```python
from build123d import *

# Parameters (mm, degrees)
SKETCH1_R             = 1.60655
BOSS_EXTRUDE1_DEPTH   = 0.83
BOSS_EXTRUDE4_START   = 13.5
SKETCH3_R             = 1.5
BOSS_EXTRUDE4_DEPTH   = 0.83
BOSS_EXTRUDE5_START   = -12.67
SKETCH3_5_R           = 1.5
BOSS_EXTRUDE5_DEPTH   = 0.83
BODY_MOVE_COPY1_ANGLE = 180


with BuildPart() as part:
    # Sketch1 → Boss-Extrude1 (new body)
    with BuildSketch(Plane(origin=(0, 0, 0), x_dir=(1, 0, 0), z_dir=(0, 1, 0))):
        with BuildLine():
            Line((13.5, -4.5), (13.5, 10))
            Line((13.5, 10), (8.75, 10))
            ThreePointArc((8.75, 10), (0, 7.25), (-8.75, 10))
            Line((-8.75, 10), (-13.5, 10))
            Line((-13.5, 10), (-13.5, -4.5))
            ThreePointArc((-13.5, -4.5), (-7.288689869, -8.572238768), (0, -10))
            ThreePointArc((0, -10), (7.288689869, -8.572238768), (13.5, -4.5))
        make_face()
        with Locations(Location((-7.25, 0, 0), (0, 0, 90))):
            Circle(SKETCH1_R, mode=Mode.SUBTRACT)
        with Locations(Location((7.25, 0, 0), (0, 0, 90))):
            Circle(SKETCH1_R, mode=Mode.SUBTRACT)
    extrude(amount=BOSS_EXTRUDE1_DEPTH)

    # Sketch3 → Boss-Extrude4 (add)
    with BuildSketch(Plane(origin=(0, 0, 0), x_dir=(0, 0, -1), z_dir=(1, 0, 0)).offset(BOSS_EXTRUDE4_START)):
        with BuildLine():
            Line((-4.5, 0.83), (10, 0.83))
            Line((10, 0.83), (11.5, 0.83))
            Line((11.5, 0.83), (11.5, 2.455))
            ThreePointArc((11.5, 2.455), (16.261860542, 10.323052182), (7.082672814, 10.892326816))
            ThreePointArc((7.082672814, 10.892326816), (2.026582548, 6.580128686), (-4.5, 5.33))
            Line((-4.5, 5.33), (-4.5, 0.83))
        make_face()
        with Locations((11.5, 7.83)):
            Circle(SKETCH3_R, mode=Mode.SUBTRACT)
    extrude(amount=-BOSS_EXTRUDE4_DEPTH)

    # Sketch3<5> → Boss-Extrude5 (add)
    with BuildSketch(Plane(origin=(0, 0, 0), x_dir=(0, 0, -1), z_dir=(1, 0, 0)).offset(BOSS_EXTRUDE5_START)):
        with BuildLine():
            Line((-4.5, 0.83), (10, 0.83))
            Line((10, 0.83), (11.5, 0.83))
            Line((11.5, 0.83), (11.5, 2.455))
            ThreePointArc((11.5, 2.455), (16.261860542, 10.323052182), (7.082672814, 10.892326816))
            ThreePointArc((7.082672814, 10.892326816), (2.026582548, 6.580128686), (-4.5, 5.33))
            Line((-4.5, 5.33), (-4.5, 0.83))
        make_face()
        with Locations((11.5, 7.83)):
            Circle(SKETCH3_5_R, mode=Mode.SUBTRACT)
    extrude(amount=-BOSS_EXTRUDE5_DEPTH)

    # Fillet4
    # an asymmetric fillet: 4, 3 mm, written as the material it takes off along each edge
    with BuildSketch(Plane(origin=(-4.106690229, 5.33, 4.5), x_dir=(0, -1, 0), z_dir=(-1, 0, 0))) as fillet4_piece_1:
        with BuildLine():
            Bezier((2.727713921, 0), (0.459985745, 0), (-0.21539832, -3.418544638), weights=[1, 0.772599008, 1])
            ThreePointArc((-0.21539832, -3.418544638), (0.005386199, -1.716397689), (0, 0))
            Line((0, 0), (2.727713921, 0))
        make_face()
    extrude(amount=17.956619542, mode=Mode.SUBTRACT)

    # Fillet5
    # an asymmetric fillet: 4, 3 mm, written as the material it takes off along each edge
    with BuildSketch(Plane(origin=(22.063309771, 5.33, 4.5), x_dir=(0, -1, 0), z_dir=(-1, 0, 0))) as fillet5_piece_1:
        with BuildLine():
            Bezier((2.727713921, 0), (0.459985745, 0), (-0.21539832, -3.418544638), weights=[1, 0.772599008, 1])
            ThreePointArc((-0.21539832, -3.418544638), (0.005386199, -1.716397689), (0, 0))
            Line((0, 0), (2.727713921, 0))
        make_face()
    extrude(amount=17.956619542, mode=Mode.SUBTRACT)


with BuildPart() as part_1:
    # Body-Move/Copy1: moved
    add(part.part.moved(Location((0, 0, 0))).rotate(Axis((0, 6.6025, -3.4375), (1, 0, 0)), BODY_MOVE_COPY1_ANGLE))


solid = part_1.part
```
The model under review builds one solid part; all positions refer to its coordinate system, in mm. A direction names the side the tool comes from. Give positions to 0.01 mm unless a question says otherwise; leave off trailing zeros. Write each loop counter-clockwise with the first axis right and the second up, starting at its lowest first coordinate (ties: lowest second). Pieces come first, ordered by that corner, then holes. Notation, with made-up numbers: (-11, 49.5) - (6, 49.5) arc R13 cw to (6, 53.5) - close; hole circle Ø9 at (80, 17). An arc over 180 degrees is marked (long way). Answer in a Markdown table with one row per item. Add a question column.
1. We need section C-C on z = -6.75. Write out the cut boundary in (x, y) (3 decimals).
2. We need section B-B on x = 7.75. Write out the cut boundary in (y, z) (3 decimals), then the cut area to 3 significant figures.
3. Tool access review of faces 1 (the flat face through (-13, 12, 4.625)), 2 (the flat face through (12.67, 7, 2)), 3 (the cylindrical face through (13.09, 4.11, 5.43)): name each direction out of +Z, -Z, +X, -X, +Y, -Y from which nothing blocks a thin tool from reaching the whole face with its end or side.
4. We need section D-D on y = 2.75. Write out the cut boundary in (x, z).
5. We need section A-A on y = 5.75. Write out the cut boundary in (x, z).
6. Draft analysis for pull direction X (two halves, no side actions). For faces 4 (the cylindrical face through (7.865, 12.796, -5.391)), 5 (the cylindrical face through (0.13, 12.796, 0.376)), 6 (the flat face through (-13.5, 8, -1)), 7 (the flat face through (-13, 11, -11.375)), state which applies: +X half, -X half, draft (parallel to the pull), parting line (faces both ways), or undercut.
7. Wall thickness on line 1 along X through (y, z) = (11.75, -6.5); line 2 along Y through (x, z) = (4, -0.5) (3 decimals); line 3 along Z through (x, y) = (-7.25, 12.9): over which ranges is each line inside the solid? List them lowest first. Write a range as [from, to].
8. Insertion check: P1, Ø0.7, axis at x = -13, z = 4, coming from the +Y side (3 decimals); P2, Ø0.7, axis at x = 13.5, y = 11.5, coming from the +Z side (3 decimals); P3, Ø6, axis at x = 2.5, y = 10, coming from the +Z side. Each pin has a flat end and moves straight along its axis. Give the tip position at first contact, or say it passes through.
Ans:
| question | item | result |
|---|---|---|
| 1 | outline | (-13.5, 7.361) - (-12.67, 7.361) - (-12.67, 12.375) - (-8.852, 12.375) - (-8.852, 13.205) - (-13.5, 13.205) - close; (-5.648, 12.375) - (5.648, 12.375) - (5.648, 13.205) - (-5.648, 13.205) - close; (8.852, 12.375) - (12.67, 12.375) - (12.67, 7.361) - (13.5, 7.361) - (13.5, 13.205) - (8.852, 13.205) - close |
| 2 | outline | (12.375, -15.252) - (13.205, -15.252) - (13.205, -8.402) - (12.375, -8.402) - close; (12.375, -5.348) - (13.205, -5.348) - (13.205, 2.484) - (12.375, 2.484) - close |
| 2 | area | 12.2 mm^2 |
| 3 | face 1 | +Z, +X, -X, +Y |
| 3 | face 2 | +Z, -Z, -Y |
| 3 | face 3 | +X, -X |
| 4 | outline | (-13.5, -0.11) - (-12.67, -0.11) - (-12.67, 9.32) - (-13.5, 9.32) - close; (12.67, -0.11) - (13.5, -0.11) - (13.5, 9.32) - (12.67, 9.32) - close |
| 5 | outline | (-13.5, -3.31) - (-12.67, -3.31) - (-12.67, 3.17) - (-13.5, 3.17) - close; (-13.5, 6.08) - (-12.67, 6.08) - (-12.67, 9.99) - (-13.5, 9.99) - close; (12.67, -3.31) - (13.5, -3.31) - (13.5, 3.17) - (12.67, 3.17) - close; (12.67, 6.08) - (13.5, 6.08) - (13.5, 9.99) - (12.67, 9.99) - close |
| 6 | face 4 | undercut |
| 6 | face 5 | undercut |
| 6 | face 6 | -X half |
| 6 | face 7 | draft |
| 7 | line 1 | x = [-13.5, -12.67], [12.67, 13.5] |
| 7 | line 2 | y = [12.375, 13.205] |
| 7 | line 3 | z = [-15.46, -8.48], [-5.27, 2.2] |
| 8 | P1 | stops at y = 12.375 |
| 8 | P2 | stops at z = 4.625 |
| 8 | P3 | stops at z = 1 |
